The listing builds one solid part. Answer for the finished solid, in the listing's coordinates (mm). A direction names the side the tool comes from. Coordinates: 2 decimals unless noted, no trailing zeros. Order: outer loops, then holes, each group sorted by start corner. A loop starts at its lowest first (then second) coordinate and runs counter-clockwise, first axis right, second up. Notation, with made-up numbers: (-6.75, -5) -> (37.25, -5) arc R30 cw to (37.25, 19) -> close; hole circle Ø4 at (-22, 82). An arc over 180 degrees is marked (long way). Answer in a Markdown table with one row per item.
Autodesk Inventor part; units mm, degrees
ref_plane "YZ Plane" through (0, 0, 0) normal (1, 0, 0) x (0, 1, 0)
ref_plane "XZ Plane" through (0, 0, 0) normal (0, 1, 0) x (-1, 0, 0)
ref_plane "XY Plane" through (0, 0, 0) normal (0, 0, 1) x (1, 0, 0)
sketch "Sketch1" plane through (0, 0, 0) normal (0, 1, 0) x (-1, 0, 0)
  line L0 (0, 0) -> (485, 0)
  line L1 (485, 0) -> (485, -415)
  line L2 (485, -415) -> (0, -415)
  line L3 (0, -415) -> (0, 0)
  line L4 (0, 0) -> (25, 0)
  line L5 (25, 0) -> (25, -415)
  line L6 (25, -415) -> (0, -415)
  line L7 (0, -415) -> (0, 0)
  line L8 (25, 0) -> (300, 0)
  line L9 (300, 0) -> (300, -75)
  line L10 (300, -75) -> (25, -75)
  line L11 (25, -75) -> (25, 0)
  line L12 (25, -415) -> (300, -415)
  line L13 (300, -415) -> (300, -340)
  line L14 (300, -340) -> (25, -340)
  line L15 (25, -340) -> (25, -415)
  line L16 (25, -207.5) -> (400, -207.5)
  arc A0 (300, -340) -> (300, -75) centre (262.2188, -207.5) ccw
  point P0 (25, -340)
  point P1 (25, -75)
  dimension "d0" = 485
  dimension "d1" = 415
  dimension "d2" = 25
  dimension "d3" = 275
  dimension "d4" = 75
  dimension "d5" = 275
  dimension "d6" = 75
  dimension "d7" = 375
extrude "Extrusion1" add sketch "Sketch1" along normal blind 5 contours L0 L5 L2 L3 | L0 L9 L10 L5 | L0 L1 L2 L13 A0 L9 | L5 L14 L13 L2
fillet "Fillet1" radius 25 4 edges at (-25, 2.5, -340) (-25, 2.5, -75) (-300, 2.5, -75) (-300, 2.5, -340)
sketch "Sketch2" plane through (-485, 0, 0) normal (0, 0, 1) x (1, 0, 0)
  line L0 (0, 0) -> (485, 0)
  line L1 (0, 5) -> (485, 5)
  line L2 (0, 0) -> (485, 0)
  line L3 (485, 0) -> (485, 5)
  line L4 (485, 5) -> (0, 5)
  line L5 (0, 5) -> (0, 0)
extrude "Extrusion2" add sketch "Sketch2" along normal blind 10
sketch "Sketch3" plane through (0, 0, -415) normal (0, 0, -1) x (-1, 0, 0)
  line L0 (485, 0) -> (485, 5)
  line L1 (485, 5) -> (0, 5)
  line L2 (0, 5) -> (0, 0)
  line L3 (0, 0) -> (485, 0)
  line L4 (485, 0) -> (485, 5)
extrude "Extrusion3" add sketch "Sketch3" along normal blind 10
sketch "Sketch4" plane through (0, 5, 0) normal (0, 1, 0) x (1, 0, 0)
  line L0 (0, 0) -> (-242.5, 0)
  line L1 (-242.5, 0) -> (-242.5, 4.5)
  line L2 (-242.5, 4.5) -> (0, 4.5)
  line L3 (0, 4.5) -> (0, 0)
  line L4 (-485, -10) -> (-485, 425)
  line L5 (-485, 425) -> (-485, 415)
  line L6 (-485, 415) -> (-242.5, 415)
  line L7 (-242.5, 415) -> (-242.5, 410.5)
  line L8 (-242.5, 410.5) -> (-485, 410.5)
  line L9 (-485, 410.5) -> (-485, 415)
  line L10 (0, 425) -> (0, -10)
  dimension "d15" = 4.5
  dimension "d16" = 4.5
  dimension "d17" = 242.5
  dimension "d18" = 10
  dimension "d19" = 4.5
  dimension "d20" = 242.5
extrude "Extrusion4" cut sketch "Sketch4" against normal blind 5
sketch "Sketch6" plane through (0, 5, 0) normal (0, 1, 0) x (1, 0, 0)
  line L0 (-485, 410.5) -> (-485, 202.5446)
  line L1 (-485, 410.5) -> (-485, 362)
  line L2 (-485, 362) -> (-470, 362)
  line L3 (-470, 362) -> (-470, 366.5)
  line L4 (-470, 366.5) -> (-485, 366.5)
  line L5 (-485, 366.5) -> (-485, 362)
  line L6 (-485, 309.75) -> (-470, 309.75)
  line L7 (-470, 309.75) -> (-470, 314.25)
  line L8 (-470, 314.25) -> (-485, 314.25)
  line L9 (-485, 314.25) -> (-485, 309.75)
  line L10 (-485, 257.5) -> (-470, 257.5)
  line L11 (-470, 257.5) -> (-470, 262)
  line L12 (-470, 262) -> (-485, 262)
  line L13 (-485, 262) -> (-485, 257.5)
  line L14 (-485, 205.25) -> (-470, 205.25)
  line L15 (-470, 205.25) -> (-470, 209.75)
  line L16 (-470, 209.75) -> (-485, 209.75)
  line L17 (-485, 209.75) -> (-485, 205.25)
  line L18 (-485, 153) -> (-470, 153)
  line L19 (-470, 153) -> (-470, 157.5)
  line L20 (-470, 157.5) -> (-485, 157.5)
  line L21 (-485, 157.5) -> (-485, 153)
  line L22 (-485, 100.75) -> (-470, 100.75)
  line L23 (-470, 100.75) -> (-470, 105.25)
  line L24 (-470, 105.25) -> (-485, 105.25)
  line L25 (-485, 105.25) -> (-485, 100.75)
  line L26 (-485, 48.5) -> (-470, 48.5)
  line L27 (-470, 48.5) -> (-470, 53)
  line L28 (-470, 53) -> (-485, 53)
  line L29 (-485, 53) -> (-485, 48.5)
  line L30 (-485, -10) -> (-485, 410.5)
  line L31 (-485, 410.5) -> (-452.1188, 410.5)
  line L32 (-242.5, 410.5) -> (-485, 410.5)
  point P0 (0, 0)
  dimension "d27" = 48.5
  dimension "d28" = 15
  dimension "d29" = 4.5
  dimension "d30" = 52.25
  dimension "d32" = 0
extrude "Extrusion5" cut sketch "Sketch6" against normal blind 5 contours L4 L3 L2 L0 | L28 L27 L26 L29 | L24 L23 L22 L25 | L20 L19 L18 L21 | L12 L11 L10 L0 | L8 L7 L6 L0
ref_plane "Work Plane1" through (0, 5, -430.1373) normal (0, 0, -1) x (-1, 0, 0)
fillet "Fillet2" radius 1 32 edges at (-242.5, 2.5, 0) (-242.5, 2.5, -4.5) (0, 2.5, 0) (0, 2.5, -4.5) (-470, 2.5, -48.5) (-470, 2.5, -53) (-485, 2.5, -53) (-485, 2.5, -48.5) (-470, 2.5, -100.75) (-470, 2.5, -105.25) (-485, 2.5, -105.25) (-485, 2.5, -100.75) (-485, 2.5, -157.5) (-485, 2.5, -153) (-470, 2.5, -153) (-470, 2.5, -157.5) (-485, 2.5, -257.5) (-470, 2.5, -257.5) (-470, 2.5, -262) (-485, 2.5, -262) (-470, 2.5, -309.75) (-470, 2.5, -314.25) (-485, 2.5, -314.25) (-485, 2.5, -309.75) (-485, 2.5, -366.5) (-485, 2.5, -362) (-470, 2.5, -362) (-470, 2.5, -366.5) (-485, 2.5, -410.5) (-485, 2.5, -415) (-242.5, 2.5, -410.5) (-242.5, 2.5, -415)
sketch "Sketch10" plane through (-485, 0, -409.5) normal (-1, 0, 0) x (0, 0, 1)
  line L0 (42, 5) -> (0, 5)
  line L1 (21, 5) -> (21, 0)
  line L2 (21, 0) -> (11, 0)
  line L3 (0, 0) -> (42, 0)
  line L4 (11, 0) -> (31, 0)
  line L5 (31, 0) -> (31, 5)
  line L6 (31, 5) -> (11, 5)
  line L7 (11, 5) -> (11, 0)
  line L8 (70.6707, 5) -> (333.3293, 5)
  line L9 (202, 5) -> (202, -36.8909)
  line L10 (383, 5) -> (383, 0)
  line L11 (383, 0) -> (393, 0)
  line L12 (393, 0) -> (373, 0)
  line L13 (373, 0) -> (373, 5)
  line L14 (373, 5) -> (393, 5)
  line L15 (393, 5) -> (393, 0)
  point P0 (409.5, 0)
  point P1 (31, 0)
  point P2 (11, 5)
  dimension "d44" = 10
  dimension "d45" = 20
extrude "Extrusion9" add sketch "Sketch10" along normal blind 5 contours L1 L2 L7 L0 | L14 L15 L11 L10
sketch "Sketch12" plane through (0, 5, 0) normal (0, 1, 0) x (1, 0, 0)
  line L0 (0, -10) -> (-485, -10)
  line L1 (-485, -10) -> (-485, -15)
  line L2 (-485, -15) -> (0, -15)
  line L3 (0, -15) -> (0, -10)
  line L4 (0, 425) -> (-485, 425)
  line L5 (-485, 425) -> (0, 425)
  line L6 (0, 425) -> (0, 430)
  line L7 (0, 430) -> (-485, 430)
  line L8 (-485, 430) -> (-485, 425)
  point P0 (0, 0)
  dimension "d48" = 5
  dimension "d49" = 5
extrude "Extrusion10" add sketch "Sketch12" against normal blind 5
properties part number "outside_leg" material "Foam Core Board"
(1) A cutting plane is placed at D-D, the plane x = -31.5. Determine the outline of the cut face in (y, z), then the cut area to 3 significant figures.
Check values:
| item | result |
|---|---|
| outline | (0, -430) -> (5, -430) -> (5, -331.82) -> (0, -331.82) -> close; (0, -83.18) -> (5, -83.18) -> (5, -4.5) -> (0, -4.5) -> close; (0, 0) -> (5, 0) -> (5, 15) -> (0, 15) -> close |
| area | 959 mm² |
(2) Find the intervals of material crossed by line 1 along Z through (x, y) = (-274, 3.85); line 2 along Z through (x, y) = (-340, 3.8); line 3 along Z through (x, y) = (-21.5, 3.3), in increasing order. Write a range as from..to.
Check values:
| item | result |
|---|---|
| line 1 | -430..-415, -410.5..-340, -75..15 |
| line 2 | -430..-415, -410.5..-321.23, -93.77..15 |
| line 3 | -430..-4.5, 0..15 |
(3) Flat-ended cylindrical pins translate along their axes: pin 1 (3 mm diameter, centred on y = 4, z = -178.5, fed in from -X); pin 2 (2 mm diameter, centred on y = 2, z = -311.5, fed in from -X); pin 3 (3 mm diameter, centred on y = 1.5, z = -51, fed in from -X). Find the tip coordinate at first contact, or state that the pin passes through.
Check values:
| item | result |
|---|---|
| pin 1 | x = -485 |
| pin 2 | x = -470.03 |
| pin 3 | x = -470.13 |
(4) For a pull along Z with two mould halves and no side action, classify faces 3 (the cylindrical face through (-399.98, 2.46, -205.06)), 4 (the flat face through (-405, 0, -204)) as released by +Z, released by -Z, zero draft, split by the parting line, or undercut.
Check values:
| item | result |
|---|---|
| face 3 | undercut |
| face 4 | zero draft |
(5) A cutting plane is placed at B-B, the plane z = -193.5. Determine the outline of the cut face in (x, y), then the cut area to 3 significant figures.
Check values:
| item | result |
|---|---|
| outline | (-485, 0) -> (-399.29, 0) -> (-399.29, 5) -> (-485, 5) -> close; (-25, 0) -> (0, 0) -> (0, 5) -> (-25, 5) -> close |
| area | 554 mm² |
(6) A cutting plane is placed at C-C, the plane z = -238. Determine the outline of the cut face in (x, y).
Check values:
| item | result |
|---|---|
| outline | (-485, 0) -> (-396.58, 0) -> (-396.58, 5) -> (-485, 5) -> close; (-25, 0) -> (0, 0) -> (0, 5) -> (-25, 5) -> close |
(7) A cutting plane is placed at A-A, the plane x = -101. Determine the outline of the cut face in (y, z).
Check values:
| item | result |
|---|---|
| outline | (0, -430) -> (5, -430) -> (5, -340) -> (0, -340) -> close; (0, -75) -> (5, -75) -> (5, -4.5) -> (0, -4.5) -> close; (0, 0) -> (5, 0) -> (5, 15) -> (0, 15) -> close |
(8) Which of the six approach directions +Z, -Z, +X, -X, +Y, -Y give full straight-line access (tool end or side, diameter ignored) to faces 1 (the flat face through (-357, 5, -105)), 2 (the cylindrical face through (-32.129, 2.535, -332.482))?
Check values:
| item | result |
|---|---|
| face 1 | +Z, -Z, +X, -X, +Y |
| face 2 | +Y, -Y |
